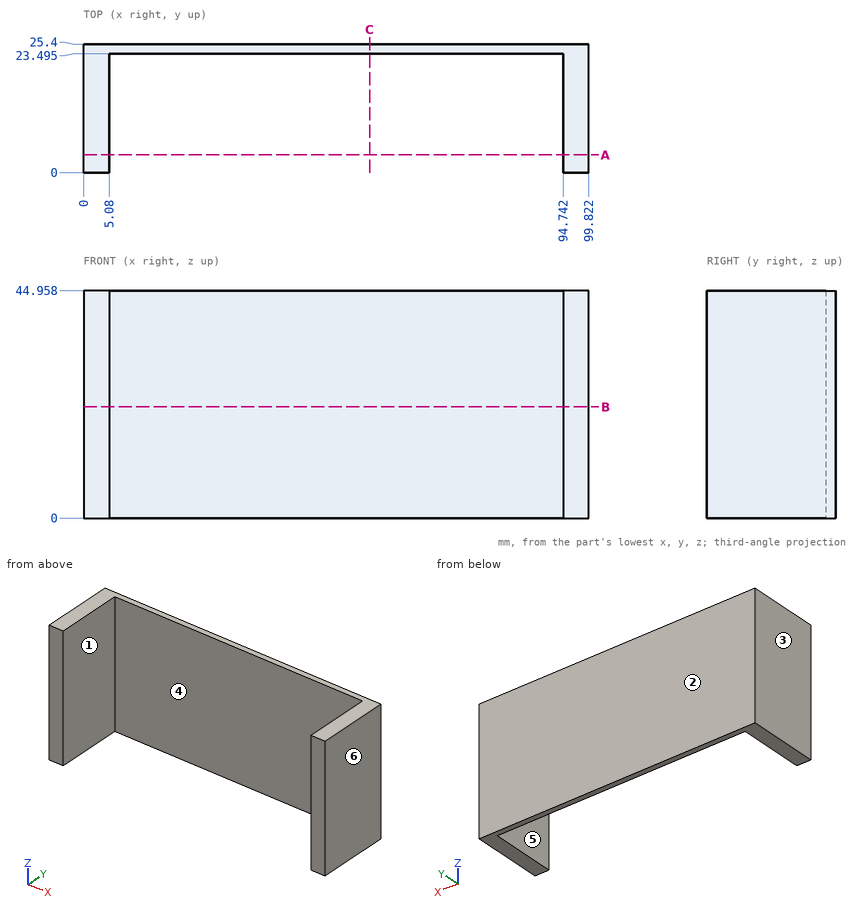
Input: dimensioned drawing with shaded views. Units: mm. Origin: part minimum x, y, z. A direction names the side the tool comes from. Give positions to 0.01 mm unless a question says otherwise; leave off trailing zeros. Write each loop counter-clockwise with the first axis right and the second up, starting at its lowest first coordinate (ties: lowest second). Pieces come first, ordered by that corner, then holes.
Q1. Section C-C, the plane x = 56.5. Output: boundary loops of the cut face in (y, z) (3 decimals).
Q2. Material intervals for probe 1 along X at (y, z) = (13, 15); probe 2 along Y at (x, z) = (84, 30) (3 decimals), sorted ascending.
Q3. Section B-B, the plane z = 22. Output: boundary loops of the cut face in (x, y) (3 decimals).
Q4. Pull-direction query (X, two-part tool) for the marked faces 1, 2, 3 and 4; classes: pulls with the +X half, pulls with the -X half, needs draft (parallel to the pull), parting line crosses it, or undercut.
Q5. Set-up query: the marked faces 5 and 6. Return all of +Z, -Z, +X, -X, +Y, -Y with unobstructed straight access to the full face (end or side cutting, diameter ignored); none if empty.
Q6. Section A-A, the plane y = 3.5. Output: boundary loops of the cut face in (x, z), plus the area to 3 significant figures.
Q7. First-contact query: P1, Ø12, axis at x = 41, y = 19, coming from the +Z side. Flat tip, straight axial feed; report the tip coordinate or a pass-through.
Filled in:
1. outline: (23.495, 0) - (25.4, 0) - (25.4, 44.958) - (23.495, 44.958) - close
2. probe 1: x = 0 to 5.08, 94.74 to 99.82
2. probe 2: y = 23.495 to 25.4
3. outline: (0, 0) - (5.08, 0) - (5.08, 23.495) - (94.742, 23.495) - (94.742, 0) - (99.822, 0) - (99.822, 25.4) - (0, 25.4) - close
4. face 1: undercut
4. face 2: needs draft
4. face 3: pulls with the -X half
4. face 4: undercut
5. face 5: +Z, -Z, -Y
5. face 6: +Z, -Z, +X, +Y, -Y
6. outline: (0, 0) - (5.08, 0) - (5.08, 44.96) - (0, 44.96) - close; (94.74, 0) - (99.82, 0) - (99.82, 44.96) - (94.74, 44.96) - close
6. area: 457 mm2
7. P1: stops at z = 44.96
